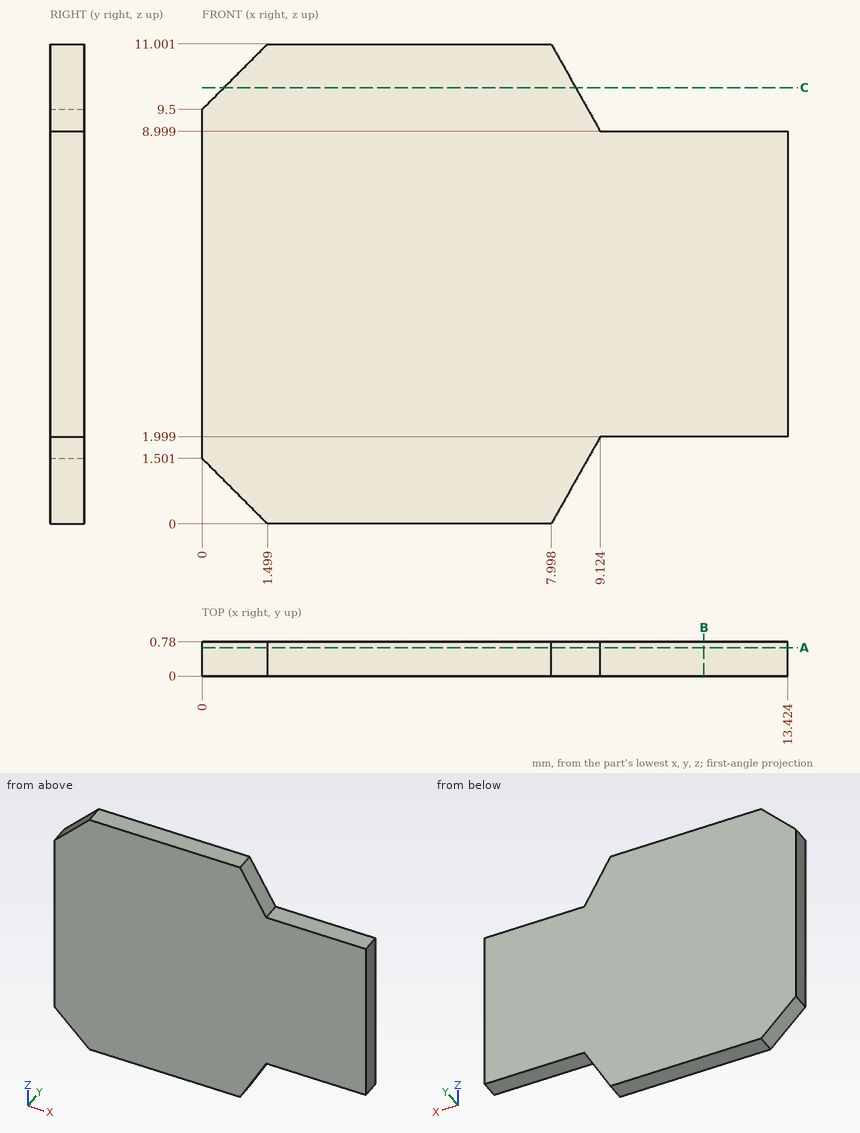
Check sheet for the drawn part. Datum: minimum x, y, z corner. Units: mm. Give positions to 0.01 mm unless a question says otherwise; leave off trailing zeros. Write each loop counter-clockwise with the first axis right and the second up, starting at its lowest first coordinate (ties: lowest second). Pieces come first, ordered by that corner, then holes. Notation, with made-up numbers: (-6.75, 86) -> (51.25, 86) arc R20 ccw to (51.25, 118) -> close; hole circle Ø1 at (11.5, 55.25). An arc over 180 degrees is marked (long way). Use one line per item in the form item = value. Start each with the question number.
1. Section check C-C (z = 10). Record the cut outline in (x, y).
2. Section check A-A (y = 0.65). Record the cut outline in (x, z), and give its area (3 significant figures).
3. Section check B-B (x = 11.5). Record the cut outline in (y, z).
4. Thickness scan on line 1 along Z through (x, y) = (10, 0.6). Record the ranges inside material, lowest first. Write a range as from..to.
Conclusion:
q1.outline = (0.5, 0) -> (8.56, 0) -> (8.56, 0.78) -> (0.5, 0.78) -> close
q2.outline = (0, 1.5) -> (1.5, 0) -> (8, 0) -> (9.12, 2) -> (13.42, 2) -> (13.42, 9) -> (9.12, 9) -> (8, 11) -> (1.5, 11) -> (0, 9.5) -> close
q2.area = 126 mm²
q3.outline = (0, 2) -> (0.78, 2) -> (0.78, 9) -> (0, 9) -> close
q4.line_1 = 2..9
